Model file for the job. Use its own axes, mm. A direction names the side the tool comes from. Round coordinates to 2 decimals unless told otherwise and drop trailing zeros. Order: outer loops, then holes, each group sorted by start corner. A loop starts at its lowest first (then second) coordinate and runs counter-clockwise, first axis right, second up. Notation, with made-up numbers: (-25, 32.5) - (22, 32.5) arc R27 ccw to (22, 63.5) - close; hole circle Ø1 at (-27.75, -12.75). An arc over 180 degrees is marked (long way). Put each result on its own line as item: value. Start each with the question number.
Item 1: Saw through at D-D on x = 0. List the corners of the cut face in (y, z), plus the area to 3 significant figures.
Item 2: Probe probe 1 along Y at (x, z) = (-1.75, -1.75); probe 2 along Y at (x, z) = (-0.75, -3.5); probe 3 along X at (y, z) = (-2, 0). List the from-to ranges inside material, lowest first.
Item 3: Saw through at B-B on x = 1.5. List the corners of the cut face in (y, z).
Item 4: Saw through at A-A on z = 0. List the corners of the cut face in (x, y).
Item 5: Mould opens along X. For faces 1 (the face through (2, 3, 0)), 2 (the face through (2, -10, 0)), 3 (the face through (1, 2, 0)) say: pulls with the +X half, pulls with the -X half, needs draft (parallel to the pull), parting line crosses it, or undercut.
Item 6: Pin check, flat tips, straight feed: pin 1 Ø1 at (x, y) = (-3, -15) entering from -Z; pin 2 Ø3 at (y, z) = (-15.5, 2.5) entering from -X; pin 3 Ø1.5 at (y, z) = (-2, 2) entering from +X; pin 4 Ø1.6 at (x, z) = (0, 0) entering from +Y. Stop position of each tip, or through.
Item 7: Which spindle directions (+Z, -Z, +X, -X, +Y, -Y) get a long thin tool onto all of the face, cutting with end or side? Do faces 4 (the face through (0, 1.5, 0)), 5 (the face through (-1, 0, -2)), 6 (the face through (0, -20, 0)). Say none if no direction does.
Item 8: Saw through at C-C on y = -2.75. List the corners of the cut face in (x, z), plus the area to 3 significant figures.
```python
from build123d import *

# Parameters (mm, degrees)
SKETCH1_R          = 4
EXTRUDE1_DEPTH     = 3
CUT_EXTRUDE1_DEPTH = 1.5
SKETCH3_R          = 2
EXTRUDE2_DEPTH     = 20


with BuildPart() as part:
    # Sketch1 → Extrude1 (new body)
    with BuildSketch(Plane(origin=(0, 0, 0), x_dir=(1, 0, 0), z_dir=(0, 1, 0))):
        with Locations(Location((0, 0, 0), (0, 0, 270))):  # turned: the seam where the file's is
            Circle(SKETCH1_R)
    extrude(amount=EXTRUDE1_DEPTH)

    # Sketch2 → Cut-Extrude1 (cut)
    with BuildSketch(Plane(origin=(0, 3, 0), x_dir=(-1, 0, 0), z_dir=(0, 1, 0))):
        Polygon((0, 4.401224563), (-1, 4.401224563), (-1, -5.078336035), (1, -5.078336035), (1, 4.401224563), align=None)
    extrude(amount=-CUT_EXTRUDE1_DEPTH, mode=Mode.SUBTRACT)

    # Sketch3 → Extrude2 (add)
    with BuildSketch(Plane.XZ):
        with Locations(Location((0, 0, 0), (0, 0, 90))):  # turned: the seam where the file's is
            Circle(SKETCH3_R)
    extrude(amount=EXTRUDE2_DEPTH)


solid = part.part
```
Results found:
1. outline: (-20, -2) - (0, -2) - (0, -4) - (1.5, -4) - (1.5, 4) - (0, 4) - (0, 2) - (-20, 2) - close
1. area: 92.0 mm²
2. probe 1: y = 0 to 3
2. probe 2: y = 0 to 1.5
2. probe 3: x = -2 to 2
3. outline: (-20, -1.32) - (0, -1.32) - (0, -3.71) - (3, -3.71) - (3, 3.71) - (0, 3.71) - (0, 1.32) - (-20, 1.32) - close
4. outline: (-4, 0) - (-2, 0) - (-2, -20) - (2, -20) - (2, 0) - (4, 0) - (4, 3) - (1, 3) - (1, 1.5) - (-1, 1.5) - (-1, 3) - (-4, 3) - close
5. face 1: needs draft
5. face 2: parting line crosses it
5. face 3: undercut
6. pin 1: passes through
6. pin 2: stops at x = -1.73
6. pin 3: stops at x = 1.56
6. pin 4: stops at y = 1.5
7. face 4: +Z, -Z, +Y
7. face 5: -Y
7. face 6: +Z, -Z, +X, -X, -Y
8. outline: circle Ø4 at (0, 0)
8. area: 12.6 mm²
